Here's the drawing with two shaded views (mm, measured from the low corner). I have some questions. Round coordinates to 2 decimals unless told otherwise and drop trailing zeros. Loops run counter-clockwise (first coordinate to the right, second up) from the corner with the lowest first, then second, coordinate; pieces in that order, holes last. Notation, with made-up numbers: (77, -26.75) -> (111, -26.75) arc R27 ccw to (111, -10.75) -> close; hole circle Ø9 at (37.5, 44.25). An arc over 180 degrees is marked (long way). Write item = value, one per line.
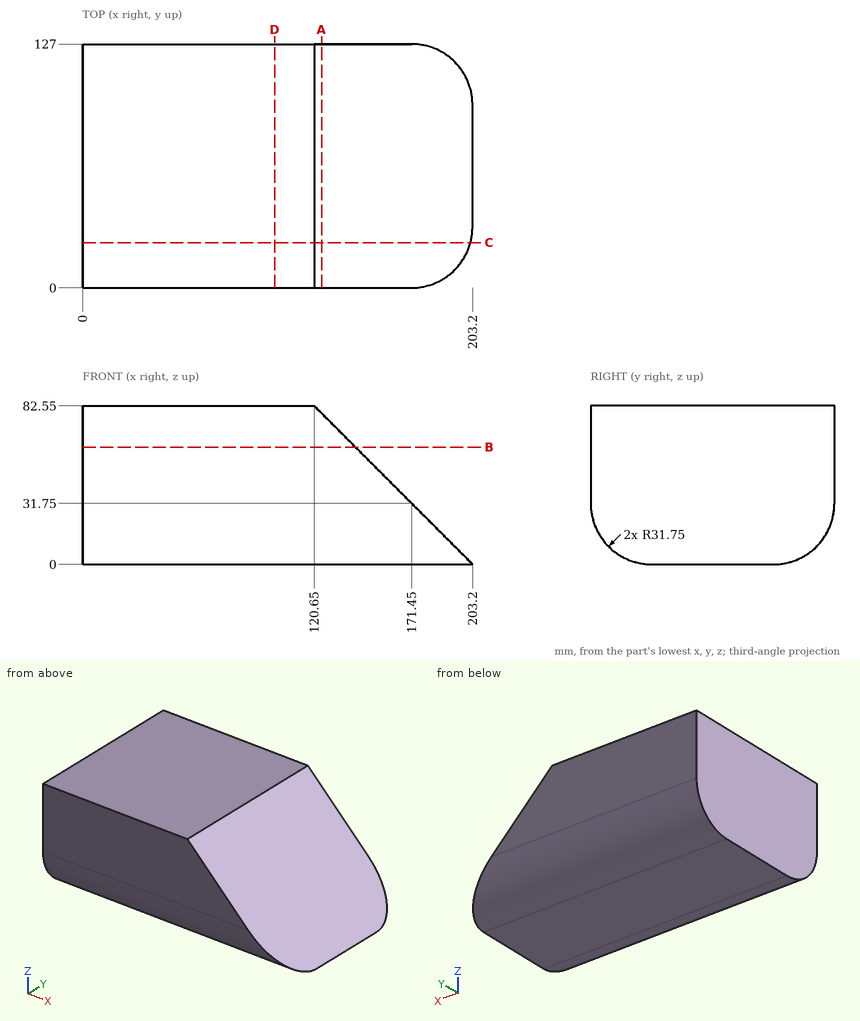
1. Suppose I cut it at D-D, the plane x = 100. List the corners of the cut face in (y, z) for me.
Entries:
outline = (0, 31.75) arc R31.75 ccw to (31.75, 0) -> (95.25, 0) arc R31.75 ccw to (127, 31.75) -> (127, 82.55) -> (0, 82.55) -> close
2. Suppose I cut it at C-C, the plane y = 23.5. List the corners of the cut face in (x, z) for me, and give its area (3 significant figures).
Entries:
outline = (0, 1.09) -> (202.11, 1.09) -> (120.65, 82.55) -> (0, 82.55) -> close
area = 13,100 mm²
3. I need wall thicknesses on line 1 (X direction, y = 28, z = 9); line 2 (X direction, y = 116, z = 78); line 3 (Y direction, x = 171.5, z = 12). Which ranges of each line are inside material? Lowest first, please. Write a range as [from, to].
Entries:
line_1 = [0, 194.2]
line_2 = [0, 125.2]
line_3 = [6.89, 120.11]
4. Suppose I cut it at A-A, the plane x = 124.5. List the corners of the cut face in (y, z) for me.
Entries:
outline = (0, 31.75) arc R31.75 ccw to (31.75, 0) -> (95.25, 0) arc R31.75 ccw to (127, 31.75) -> (127, 78.7) -> (0, 78.7) -> close
5. I'm going to push flat-ended pins straight in: pin 1 (4 mm diameter, centred on x = 91, z = 29, fed in from +Y); pin 2 (3 mm diameter, centred on y = 39, z = 10.5, fed in from +X). Where does each tip first touch, or does it pass through?
Entries:
pin_1 = 126.99
pin_2 = 194.2
6. Suppose I cut it at B-B, the plane z = 61. List the corners of the cut face in (x, y) for me, and give its area (3 significant figures).
Entries:
outline = (0, 0) -> (142.2, 0) -> (142.2, 127) -> (0, 127) -> close
area = 18,100 mm²
